Read the model definition and answer for the solid it produces. Units are mm, in the model's axes. Give positions to 0.01 mm unless a question says otherwise; leave off trailing zeros. Order: outer loops, then holes, each group sorted by start corner. A loop starts at its lowest first (then second) coordinate and runs counter-clockwise, first axis right, second up. Notation, with made-up numbers: (-7, 37) - (5, 37) arc R16 ccw to (5, 51) - close; hole circle Ø10 at (85, 55). An arc over 180 degrees is marked (long way). Use a Markdown table: item, result. Add a question column.
1. Consider L1, parallel to X at y = 10.5, z = 0.1; L2, parallel to Y at x = -11.5, z = 1.35; L3, parallel to X at y = 14, z = 0.45. Determine where each line is inside the solid, lowest interval first.
2. A flat-ended cylindrical pin translates along its axis: P1, Ø0.5, axis at y = 14, z = 1, coming from the -X side. Find the tip coordinate at first contact, or state that the pin passes through.
3. A cutting plane is placed at C-C on x = 2. Determine the outline of the cut face in (y, z), and give its area (3 significant figures).
4. A cutting plane is placed at B-B on z = 0.35. Determine the outline of the cut face in (x, y).
5. A cutting plane is placed at A-A on y = 8. Determine the outline of the cut face in (x, z).
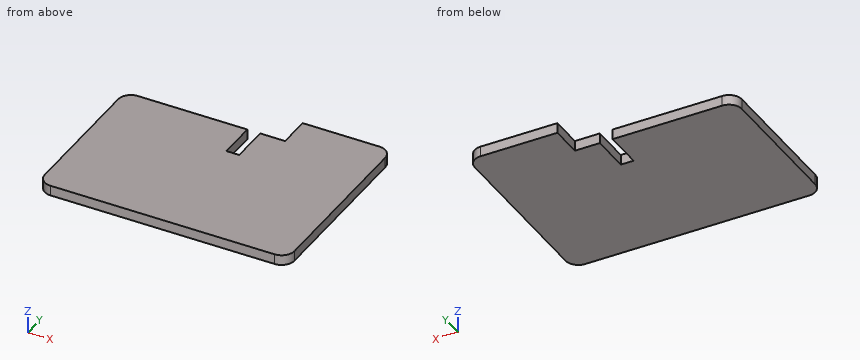
Autodesk Inventor part; units mm, degrees
ref_plane "YZ Plane" through (0, 0, 0) normal (1, 0, 0) x (0, 1, 0)
ref_plane "XZ Plane" through (0, 0, 0) normal (0, 1, 0) x (-1, 0, 0)
ref_plane "XY Plane" through (0, 0, 0) normal (0, 0, 1) x (1, 0, 0)
sketch "Sketch5" plane through (0, 0, 0) normal (0, 0, 1) x (1, 0, 0)
  line L0 (19.5002, -12.5002) -> (-19.5002, -12.5002)
  line L1 (-19.5002, -12.5002) -> (-19.5002, 12.5002)
  line L2 (19.5002, 12.5002) -> (19.5002, -12.5002)
  line L3 (19.5002, -12.5002) -> (-19.5002, 12.5002) construction
  line L4 (-19.5002, -12.5002) -> (19.5002, 12.5002) construction
  line L5 (1.6, 6.4998) -> (-0.4, 6.4998)
  line L6 (-0.4, 6.4998) -> (-0.4, 12.5002)
  line L7 (1.6, 12.5002) -> (1.6, 6.4998)
  line L8 (1.6, 6.4998) -> (-0.4, 12.5002) construction
  line L9 (-0.4, 6.4998) -> (1.6, 12.5002) construction
  line L10 (5.4998, 12.5002) -> (5.4998, 17.5003)
  line L11 (5.4998, 17.5003) -> (19.5002, 17.5003)
  line L12 (19.5002, 17.5003) -> (19.5002, 12.5002)
  line L13 (-19.5002, 12.5002) -> (-0.4, 12.5002)
  line L14 (1.6, 12.5002) -> (5.4998, 12.5002)
extrude "Extrusion4" add sketch "Sketch5" along normal blind 1.6
fillet "Fillet4" radius 2 4 edges at (19.5002, 17.5003, 0.8) (-19.5002, 12.5002, 0.8) (19.5002, -12.5002, 0.8) (-19.5002, -12.5002, 0.8)
properties part number "pcb_balun_bottom"
Output values:
| question | item | result |
|---|---|---|
| 1 | L1 | -19.5 to -0.4, 1.6 to 19.5 |
| 1 | L2 | -12.5 to 12.5 |
| 1 | L3 | 5.5 to 19.5 |
| 2 | P1 | x = 5.5 |
| 3 | outline | (-12.5, 0) - (12.5, 0) - (12.5, 1.6) - (-12.5, 1.6) - close |
| 3 | area | 40.0 mm² |
| 4 | outline | (-19.5, -10.5) arc R2 ccw to (-17.5, -12.5) - (17.5, -12.5) arc R2 ccw to (19.5, -10.5) - (19.5, 15.5) arc R2 ccw to (17.5, 17.5) - (5.5, 17.5) - (5.5, 12.5) - (1.6, 12.5) - (1.6, 6.5) - (-0.4, 6.5) - (-0.4, 12.5) - (-17.5, 12.5) arc R2 ccw to (-19.5, 10.5) - close |
| 5 | outline | (-19.5, 0) - (-0.4, 0) - (-0.4, 1.6) - (-19.5, 1.6) - close; (1.6, 0) - (19.5, 0) - (19.5, 1.6) - (1.6, 1.6) - close |
